```python
from build123d import *

# Parameters (mm, degrees)
SKETCH1_R           = 22.225
BOSS_EXTRUDE1_DEPTH = 19.05


with BuildPart() as part:
    # Sketch1 → Boss-Extrude1 (new body)
    with BuildSketch(Plane(origin=(0, 0, 0), x_dir=(0, 0, -1), z_dir=(1, 0, 0))):
        with BuildLine():
            Line((-152.4, 914.4), (-152.4, 304.8))
            ThreePointArc((-152.4, 304.8), (-226.794877579, 125.194877579), (-406.4, 50.8))
            Line((-406.4, 50.8), (-406.4, 0))
            Line((-406.4, 0), (0, 0))
            Line((0, 0), (0, 914.4))
            Line((0, 914.4), (-152.4, 914.4))
        make_face()
        with Locations(Location((-101.6, 838.2, 0), (0, 0, 180))):
            Circle(SKETCH1_R, mode=Mode.SUBTRACT)
        with Locations(Location((-38.873826797, 685.8, 0), (0, 0, 180))):
            Circle(SKETCH1_R, mode=Mode.SUBTRACT)
        with Locations(Location((-101.6, 533.4, 0), (0, 0, 180))):
            Circle(SKETCH1_R, mode=Mode.SUBTRACT)
        with Locations(Location((-38.873826797, 381, 0), (0, 0, 180))):
            Circle(SKETCH1_R, mode=Mode.SUBTRACT)
        with Locations(Location((-101.6, 228.6, 0), (0, 0, 180))):
            Circle(SKETCH1_R, mode=Mode.SUBTRACT)
    extrude(amount=BOSS_EXTRUDE1_DEPTH)


solid = part.part
```
Build history of the part. All positions in model axes, mm. Round coordinates to 2 decimals unless told otherwise and drop trailing zeros. Write each loop counter-clockwise with the first axis right and the second up, starting at its lowest first coordinate (ties: lowest second). Pieces come first, ordered by that corner, then holes.
1) Band-saw the part on C-C, the plane x = 4.75. List the corners of the cut face in (y, z) (3 decimals).
2) Band-saw the part on A-A, the plane z = 101.6. List the corners of the cut face in (x, y) (3 decimals), and give its area (3 significant figures).
3) Mould opens along Z. For faces 1 (the flat face through (9, 914.4, 75)), 2 (the flat face through (9, 614, 152.4)), 3 (the cylindrical face through (9.392, 663.764, 35.981)) say: +Z half, -Z half, draft (parallel to the pull), parting line (faces both ways), or undercut.
4) Band-saw the part on D-D, the plane y = 228.6. List the corners of the cut face in (x, z) (3 decimals), and give its area (3 significant figures).
5) Drill centre lines: probe 1 along Z at (x, y) = (7.5, 532); probe 2 along Y at (x, z) = (5.25, 47); probe 3 along Z at (x, y) = (5, 857.5). Where is each one in solid material? Low to high.
6) Band-saw the part on B-B, the plane y = 838.2. List the corners of the cut face in (x, z) (3 decimals).
7) Pin check, flat tips, straight feed: pin 1 (9.5 mm diameter, centred on x = 13, y = 695.5, fed in from +Z); pin 2 (3 mm diameter, centred on x = 16, z = 321, fed in from +Y). Stop position of each tip, or through.
Ans:
1. outline: (0, 0) - (914.4, 0) - (914.4, 152.4) - (304.8, 152.4) arc R254 cw to (50.8, 406.4) - (0, 406.4) - close; hole circle Ø44.45 at (228.6, 101.6); hole circle Ø44.45 at (381, 38.874); hole circle Ø44.45 at (533.4, 101.6); hole circle Ø44.45 at (685.8, 38.874); hole circle Ø44.45 at (838.2, 101.6)
2. outline: (0, 0) - (19.05, 0) - (19.05, 206.375) - (0, 206.375) - close; (0, 250.825) - (19.05, 250.825) - (19.05, 511.175) - (0, 511.175) - close; (0, 555.625) - (19.05, 555.625) - (19.05, 815.975) - (0, 815.975) - close; (0, 860.425) - (19.05, 860.425) - (19.05, 914.4) - (0, 914.4) - close
2. area: 14,900 mm2
3. face 1: draft
3. face 2: +Z half
3. face 3: undercut
4. outline: (0, 0) - (19.05, 0) - (19.05, 79.375) - (0, 79.375) - close; (0, 123.825) - (19.05, 123.825) - (19.05, 164.099) - (0, 164.099) - close
4. area: 2,280 mm2
5. probe 1: z = 0 to 79.42, 123.78 to 152.4
5. probe 2: y = 0 to 360.31, 401.69 to 665.11, 706.49 to 914.4
5. probe 3: z = 0 to 90.58, 112.62 to 152.4
6. outline: (0, 0) - (19.05, 0) - (19.05, 79.375) - (0, 79.375) - close; (0, 123.825) - (19.05, 123.825) - (19.05, 152.4) - (0, 152.4) - close
7. pin 1: stops at z = 152.4
7. pin 2: stops at y = 66.13
